Build history of the part. All positions in model axes, mm. Face numbers are marked on the shaded views. A direction names the side the tool comes from. Round coordinates to 2 decimals unless told otherwise and drop trailing zeros. Order: outer loops, then holes, each group sorted by start corner. A loop starts at its lowest first (then second) coordinate and runs counter-clockwise, first axis right, second up. Notation, with made-up numbers: M 81,78.5 L 120,78.5 A10 ccw 120,85.5 Z; hole C -17.75,64 d8. An arc over 180 degrees is marked long. One line per item, written item: value. Start each with the question number.
Item 1: Tool access for the marked faces 1 and 2: list every direction of +Z, -Z, +X, -X, +Y, -Y with a clear straight run to the whole face (end or side of a thin tool).
Item 2: Pin check, flat tips, straight feed: pin 1 (3 mm diameter, centred on x = 7, z = 12.5, fed in from +Y); pin 2 (2.5 mm diameter, centred on y = 9.7, z = 3.2, fed in from -X); pin 3 (1.5 mm diameter, centred on x = 7, y = 5, fed in from +Z); pin 4 (6 mm diameter, centred on x = -4, z = 9, fed in from +Y). Stop position of each tip, or through.
Item 3: Two-plate mould, pull along Y, no slides. Class the marked faces 3, 4, 5 and 6: +Y half, -Y half, draft (parallel to the pull), parting line (faces both ways), or undercut.
Item 4: Band-saw the part on A-A, the plane y = 10.5. Write the cut outline in (x, z).
Item 5: Band-saw the part on C-C, the plane y = 19. Write the cut outline in (x, z), then the cut area to 3 significant figures.
Item 6: Band-saw the part on B-B, the plane x = -2.5. Write the cut outline in (y, z) (3 decimals).
Item 7: Band-saw the part on D-D, the plane z = 10.5. Write the cut outline in (x, y), then the cut area to 3 significant figures.
Item 8: Probe L1, parallel to Y at x = -7.75, z = 3.5; L2, parallel to Z at x = -8.75, y = 14.5; L3, parallel to Z at x = -8.5, y = 8.75. List the from-to ranges inside material, lowest first.
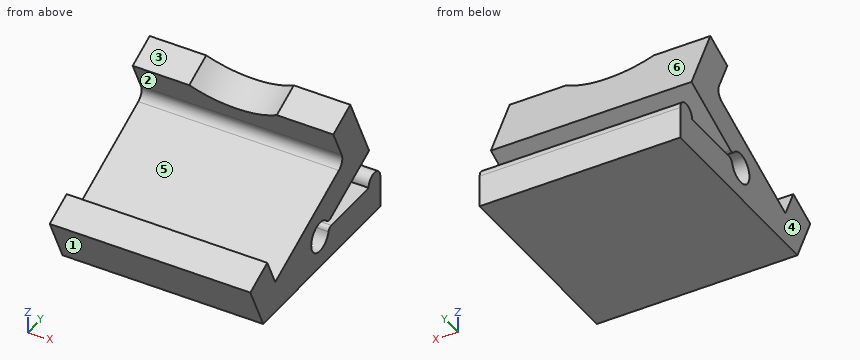
```python
from build123d import *

# Parameters (mm, degrees)
F1_DEPTH = 10
F3_DEPTH = 3.2


with BuildPart() as f1:
    # F0 (on Right) → F1 (new body, symmetric)
    with BuildSketch(Plane.YZ):
        with BuildLine():
            Line((-2.1976149611, 4.7128004926), (0, 0))
            Line((0, 0), (20, 0))
            Line((20, 0), (20, 3.2))
            ThreePointArc((20, 3.2), (19, 4.2), (18, 3.2))
            Line((18, 3.2), (11.6383557185, 3.2))
            ThreePointArc((11.6383557185, 3.2), (11.3321695007, 3.0952847075), (11.1542328002, 2.825))
            ThreePointArc((11.1542328002, 2.825), (8.2374200347, 2.8753405791), (10.8596753094, 4.1536629787))
            ThreePointArc((10.8596753094, 4.1536629787), (11.1351679799, 3.9839011426), (11.4569215283, 4.0183967448))
            Line((11.4569215283, 4.0183967448), (18.0895129826, 7.1112249333))
            Line((18.0895129826, 7.1112249333), (14.8776141934, 13.9991641148))
            Line((14.8776141934, 13.9991641148), (11.9774292749, 12.6467856772))
            Line((11.9774292749, 12.6467856772), (13.4143313648, 9.5653392013))
            ThreePointArc((13.4143313648, 9.5653392013), (13.4477161985, 8.8007007962), (12.9306418395, 8.2364131525))
            Line((12.9306418395, 8.2364131525), (2.054948395, 3.1649940116))
            Line((2.054948395, 3.1649940116), (0.7025699575, 6.0651789302))
            Line((0.7025699575, 6.0651789302), (-2.1976149611, 4.7128004926))
        make_face()
    extrude(amount=F1_DEPTH, both=True)

    # F2 (on face) → F3 (cut, through all)
    with BuildSketch(Plane(origin=(0, 14.68218615, 6.8464158402), x_dir=(1, 0, 0), z_dir=(0, -0.906307787, -0.4226182617))):
        with BuildLine():
            Line((4.3634848459, 6.4), (-4.3634848459, 6.4))
            ThreePointArc((-4.3634848459, 6.4), (0, 5), (4.3634848459, 6.4))
        make_face()
    extrude(amount=-F3_DEPTH, mode=Mode.SUBTRACT)


solid = f1.part
```
Output:
1. face 1: -Z, +X, -X, -Y
1. face 2: +X, -X, -Y
2. pin 1: stops at y = 16.28
2. pin 2: passes through
2. pin 3: stops at z = 4.89
2. pin 4: stops at y = 18.09
3. face 3: -Y half
3. face 4: draft
3. face 5: undercut
3. face 6: +Y half
4. outline: M -10,0 L 10,0 L 10,1.93 L -10,1.93 Z; M -10,4.47 L 10,4.47 L 10,7.1 L -10,7.1 Z
5. outline: M -10,0 L 10,0 L 10,4.2 L -10,4.2 Z
5. area: 84.0 mm²
6. outline: M -2.198,4.713 L 0,0 L 20,0 L 20,3.2 A1 ccw 18,3.2 L 11.638,3.2 A0.5 ccw 11.154,2.825 A1.5 cw long 10.86,4.154 A0.5 ccw 11.457,4.018 L 18.09,7.111 L 15.288,13.119 L 12.388,11.767 L 13.414,9.565 A1 cw 12.931,8.236 L 2.055,3.165 L 0.703,6.065 Z
7. outline: M -10,12.98 L 10,12.98 L 10,16.51 L -10,16.51 Z
7. area: 70.6 mm²
8. L1: y = -1.63 to 1.9, 2.77 to 8.23, 18.05 to 19.95
8. L2: z = 0 to 3.2, 5.44 to 13.82
8. L3: z = 0 to 2.04, 4.36 to 6.29
